```python
from build123d import *

# Parameters (mm, degrees)
SZKIC1_R                    = 13
SZKIC1_R_2                  = 12
SZKIC1_R_3                  = 7.5
DODANIE_WYCI_GNI_CIE1_DEPTH = 19
SFAZOWANIE1_SIZE            = 4.5
DODANIE_WYCI_GNI_CIE2_START = 19
SZKIC1_3_R                  = 16
SZKIC1_3_R_2                = 13
SZKIC1_3_R_3                = 12
SZKIC1_3_R_4                = 7.5
DODANIE_WYCI_GNI_CIE2_DEPTH = 16
DODANIE_WYCI_GNI_CIE3_START = 29
SZKIC2_R                    = 16
SZKIC2_R_2                  = 13
DODANIE_WYCI_GNI_CIE3_DEPTH = 26
DODANIE_WYCI_GNI_CIE4_START = 29
SZKIC2_3_R                  = 10
SZKIC2_3_R_2                = 7.5
DODANIE_WYCI_GNI_CIE4_DEPTH = 16
SFAZOWANIE2_SIZE            = 1.5


with BuildPart() as part:
    # Szkic1 → Dodanie-wyci_gni_cie1 (new body)
    # profile 1 of 2: a face of its own
    with BuildSketch(Plane(origin=(0, 0, 0), x_dir=(1, 0, 0), z_dir=(0, 1, 0))):
        with Locations(Location((0, 0, 0), (0, 0, 270))):
            Circle(SZKIC1_R)
        Circle(SZKIC1_R_2, mode=Mode.SUBTRACT)
    # profile 2 of 2: a face of its own
    with BuildSketch(Plane(origin=(0, 0, 0), x_dir=(1, 0, 0), z_dir=(0, 1, 0))):
        Circle(SZKIC1_R_2)
        with Locations(Location((0, 0, 0), (0, 0, 270))):
            Circle(SZKIC1_R_3, mode=Mode.SUBTRACT)
    extrude(amount=DODANIE_WYCI_GNI_CIE1_DEPTH)

    # Sfazowanie1
    sfazowanie1_edges = [part.edges().sort_by_distance(p)[0] for p in [
        (0, 0, -7.5),
    ]]
    chamfer(sfazowanie1_edges, length=SFAZOWANIE1_SIZE)

    # Szkic1_3 → Dodanie-wyci_gni_cie2 (add)
    # profile 1 of 9: a face of its own
    with BuildSketch(Plane(origin=(0, 0, 0), x_dir=(1, 0, 0), z_dir=(0, 1, 0)).offset(DODANIE_WYCI_GNI_CIE2_START)):
        Circle(SZKIC1_3_R)
        with Locations(Location((0, 0, 0), (0, 0, 270))):
            Circle(SZKIC1_3_R_2, mode=Mode.SUBTRACT)
    # profile 2 of 9: a face of its own
    with BuildSketch(Plane(origin=(0, 0, 0), x_dir=(1, 0, 0), z_dir=(0, 1, 0)).offset(DODANIE_WYCI_GNI_CIE2_START)):
        with BuildLine():
            Line((-9.237604307, 16), (-13.856406331, 8.000000225))
            ThreePointArc((-13.856406331, 8.000000225), (-7.999999911, 13.856406512), (-5.5e-08, 16))
            Line((-5.5e-08, 16), (-9.237604307, 16))
        make_face()
    # profile 3 of 9: a face of its own
    with BuildSketch(Plane(origin=(0, 0, 0), x_dir=(1, 0, 0), z_dir=(0, 1, 0)).offset(DODANIE_WYCI_GNI_CIE2_START)):
        with BuildLine():
            Line((-13.856406331, 8.000000225), (-18.475208614, 0))
            Line((-18.475208614, 0), (-13.856406442, -8.000000032))
            ThreePointArc((-13.856406442, -8.000000032), (-16, 1.11e-07), (-13.856406331, 8.000000225))
        make_face()
    # profile 4 of 9: a face of its own
    with BuildSketch(Plane(origin=(0, 0, 0), x_dir=(1, 0, 0), z_dir=(0, 1, 0)).offset(DODANIE_WYCI_GNI_CIE2_START)):
        with BuildLine():
            ThreePointArc((0, -16), (-7.999999984, -13.85640647), (-13.856406442, -8.000000032))
            Line((-13.856406442, -8.000000032), (-9.237604307, -16))
            Line((-9.237604307, -16), (0, -16))
        make_face()
    # profile 5 of 9: a face of its own
    with BuildSketch(Plane(origin=(0, 0, 0), x_dir=(1, 0, 0), z_dir=(0, 1, 0)).offset(DODANIE_WYCI_GNI_CIE2_START)):
        with BuildLine():
            ThreePointArc((13.856406442, -8.000000032), (7.999999984, -13.85640647), (0, -16))
            Line((0, -16), (9.237604307, -16))
            Line((9.237604307, -16), (13.856406442, -8.000000032))
        make_face()
    # profile 6 of 9: a face of its own
    with BuildSketch(Plane(origin=(0, 0, 0), x_dir=(1, 0, 0), z_dir=(0, 1, 0)).offset(DODANIE_WYCI_GNI_CIE2_START)):
        with BuildLine():
            ThreePointArc((16, 0), (15.454813216, -4.14110474), (13.856406442, -8.000000032))
            Line((13.856406442, -8.000000032), (18.475208614, 0))
            Line((18.475208614, 0), (13.856406447, 8.000000024))
            ThreePointArc((13.856406447, 8.000000024), (15.454813217, 4.141104735), (16, 0))
        make_face()
    # profile 7 of 9: a face of its own
    with BuildSketch(Plane(origin=(0, 0, 0), x_dir=(1, 0, 0), z_dir=(0, 1, 0)).offset(DODANIE_WYCI_GNI_CIE2_START)):
        with BuildLine():
            Line((9.237604307, 16), (-5.5e-08, 16))
            ThreePointArc((-5.5e-08, 16), (7.999999964, 13.856406481), (13.856406447, 8.000000024))
            Line((13.856406447, 8.000000024), (9.237604307, 16))
        make_face()
    # profile 8 of 9: a face of its own
    with BuildSketch(Plane(origin=(0, 0, 0), x_dir=(1, 0, 0), z_dir=(0, 1, 0)).offset(DODANIE_WYCI_GNI_CIE2_START)):
        with Locations(Location((0, 0, 0), (0, 0, 270))):
            Circle(SZKIC1_3_R_2)
        Circle(SZKIC1_3_R_3, mode=Mode.SUBTRACT)
    # profile 9 of 9: a face of its own
    with BuildSketch(Plane(origin=(0, 0, 0), x_dir=(1, 0, 0), z_dir=(0, 1, 0)).offset(DODANIE_WYCI_GNI_CIE2_START)):
        Circle(SZKIC1_3_R_3)
        with Locations(Location((0, 0, 0), (0, 0, 270))):
            Circle(SZKIC1_3_R_4, mode=Mode.SUBTRACT)
    extrude(amount=DODANIE_WYCI_GNI_CIE2_DEPTH)

    # Szkic2 → Dodanie-wyci_gni_cie3 (add)
    # profile 1 of 7: a face of its own
    with BuildSketch(Plane(origin=(0, 0, 0), x_dir=(1, 0, 0), z_dir=(0, 1, 0)).offset(DODANIE_WYCI_GNI_CIE3_START)):
        with BuildLine():
            Line((-5.5e-08, 16), (-9.237604307, 16))
            Line((-9.237604307, 16), (-13.85640621, 8.000000433))
            ThreePointArc((-13.85640621, 8.000000433), (-7.999999807, 13.856406572), (-5.5e-08, 16))
        make_face()
    # profile 2 of 7: a face of its own
    with BuildSketch(Plane(origin=(0, 0, 0), x_dir=(1, 0, 0), z_dir=(0, 1, 0)).offset(DODANIE_WYCI_GNI_CIE3_START)):
        with BuildLine():
            ThreePointArc((-13.85640621, -8.000000433), (-16, 0), (-13.85640621, 8.000000433))
            Line((-13.85640621, 8.000000433), (-18.475208614, 0))
            Line((-18.475208614, 0), (-13.85640621, -8.000000433))
        make_face()
    # profile 3 of 7: a face of its own
    with BuildSketch(Plane(origin=(0, 0, 0), x_dir=(1, 0, 0), z_dir=(0, 1, 0)).offset(DODANIE_WYCI_GNI_CIE3_START)):
        Circle(SZKIC2_R)
        with Locations(Location((0, 0, 0), (0, 0, 270))):
            Circle(SZKIC2_R_2, mode=Mode.SUBTRACT)
    # profile 4 of 7: a face of its own
    with BuildSketch(Plane(origin=(0, 0, 0), x_dir=(1, 0, 0), z_dir=(0, 1, 0)).offset(DODANIE_WYCI_GNI_CIE3_START)):
        with BuildLine():
            ThreePointArc((3.4e-08, -16), (-7.999999769, -13.856406594), (-13.85640621, -8.000000433))
            Line((-13.85640621, -8.000000433), (-9.237604307, -16))
            Line((-9.237604307, -16), (3.4e-08, -16))
        make_face()
    # profile 5 of 7: a face of its own
    with BuildSketch(Plane(origin=(0, 0, 0), x_dir=(1, 0, 0), z_dir=(0, 1, 0)).offset(DODANIE_WYCI_GNI_CIE3_START)):
        with BuildLine():
            ThreePointArc((13.856406143, -8.00000055), (7.99999974, -13.856406611), (3.4e-08, -16))
            Line((3.4e-08, -16), (9.237604307, -16))
            Line((9.237604307, -16), (13.856406143, -8.00000055))
        make_face()
    # profile 6 of 7: a face of its own
    with BuildSketch(Plane(origin=(0, 0, 0), x_dir=(1, 0, 0), z_dir=(0, 1, 0)).offset(DODANIE_WYCI_GNI_CIE3_START)):
        with BuildLine():
            Line((18.475208614, 0), (13.856406156, 8.000000528))
            ThreePointArc((13.856406156, 8.000000528), (15.454813142, 4.141105016), (16, 0))
            ThreePointArc((16, 0), (15.454813138, -4.141105028), (13.856406143, -8.00000055))
            Line((13.856406143, -8.00000055), (18.475208614, 0))
        make_face()
    # profile 7 of 7: a face of its own
    with BuildSketch(Plane(origin=(0, 0, 0), x_dir=(1, 0, 0), z_dir=(0, 1, 0)).offset(DODANIE_WYCI_GNI_CIE3_START)):
        with BuildLine():
            Line((9.237604307, 16), (-5.5e-08, 16))
            ThreePointArc((-5.5e-08, 16), (7.999999712, 13.856406627), (13.856406156, 8.000000528))
            Line((13.856406156, 8.000000528), (9.237604307, 16))
        make_face()
    extrude(amount=DODANIE_WYCI_GNI_CIE3_DEPTH)

    # Szkic2_3 → Dodanie-wyci_gni_cie4 (add)
    with BuildSketch(Plane(origin=(0, 0, 0), x_dir=(1, 0, 0), z_dir=(0, 1, 0)).offset(DODANIE_WYCI_GNI_CIE4_START)):
        with Locations(Location((0, 0, 0), (0, 0, 270))):
            Circle(SZKIC2_3_R)
        with Locations(Location((0, 0, 0), (0, 0, 270))):
            Circle(SZKIC2_3_R_2, mode=Mode.SUBTRACT)
    extrude(amount=DODANIE_WYCI_GNI_CIE4_DEPTH)

    # Sfazowanie2
    sfazowanie2_edges = [part.edges().sort_by_distance(p)[0] for p in [
        (0, 45, -10),
    ]]
    chamfer(sfazowanie2_edges, length=SFAZOWANIE2_SIZE)


solid = part.part
```
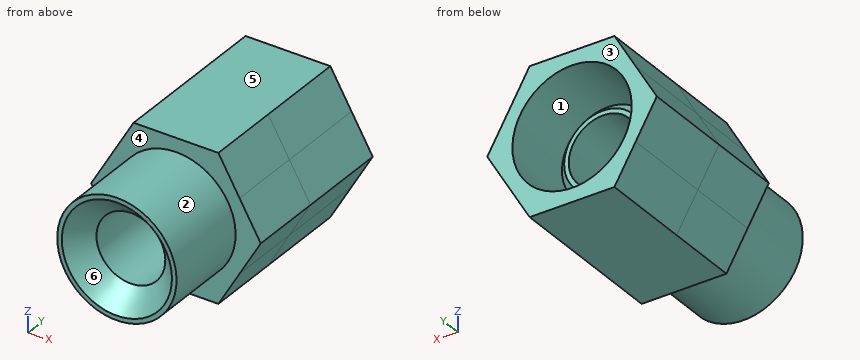
For this review, take the finished solid that the model builds, in its own axes (mm). Face numbers are marked on the shaded views. A direction names the side the tool comes from. Give positions to 0.01 mm unless a question says otherwise; leave off trailing zeros. Write each loop counter-clockwise with the first axis right and the second up, starting at its lowest first coordinate (ties: lowest second). Pieces come first, ordered by that corner, then holes.
Item 1: Take a section at C-C (x = 14.5). Give the boundary of the cut face in (y, z), and give its area (3 significant figures).
Item 2: Take a section at A-A (x = 0). Give the boundary of the cut face in (y, z), and give its area (4 significant figures).
Item 3: Insertion check: P1, Ø17, axis at x = 0, z = 0, coming from the +Y side; P2, Ø6, axis at y = 34.5, z = 8.5, coming from the -X side; P3, Ø9.5, axis at x = 0.5, z = 5, coming from the -Y side. Each pin has a flat end and moves straight along its axis. Give the tip position at first contact, or say it passes through.
Item 4: Machinability: for the marked faces 1, 2 and 3, which of the approach directions +Z, -Z, +X, -X, +Y, -Y give a long, thin tool a straight path to every point of the face, cutting with its end or side? Answer none if there is none.
Item 5: The part is to be moulded in two halves that separate along Z. For the marked faces 4, 5 and 6, say which applies: +Z half, -Z half, draft (parallel to the pull), parting line (faces both ways), or undercut.
Item 6: Wall thickness on probe 1 along X at (y, z) = (16, 0); probe 2 along X at (y, z) = (29.5, 0); probe 3 along X at (y, z) = (43, 0): over which ranges is each line inside the solid? List them lowest first.
Item 7: Take a section at B-B (y = 15). Give the boundary of the cut face in (x, z).
Established:
1. outline: (19, -6.89) - (55, -6.89) - (55, 6.89) - (19, 6.89) - close
1. area: 496 mm2
2. outline: (0, -13) - (19, -13) - (19, -16) - (55, -16) - (55, -13) - (35, -13) - (35, -10) - (43.5, -10) - (45, -8.5) - (45, -7.5) - (4.5, -7.5) - (0, -12) - close; (0, 12) - (4.5, 7.5) - (45, 7.5) - (45, 8.5) - (43.5, 10) - (35, 10) - (35, 13) - (55, 13) - (55, 16) - (19, 16) - (19, 13) - (0, 13) - close
2. area: 628.5 mm2
3. P1: stops at y = 45
3. P2: stops at x = -15.3
3. P3: stops at y = 2.23
4. face 1: +Y
4. face 2: -Y
4. face 3: +Z, -Z, +X, -X, +Y
5. face 4: draft
5. face 5: +Z half
5. face 6: undercut
6. probe 1: x = -13 to -7.5, 7.5 to 13
6. probe 2: x = -18.48 to -7.5, 7.5 to 18.48
6. probe 3: x = -18.48 to -13, -10 to -7.5, 7.5 to 10, 13 to 18.48
7. outline: circle Ø26 at (0, 0); hole circle Ø15 at (0, 0)
